For this review, take the finished solid that the model builds, in its own axes (mm). Face numbers are marked on the shaded views. A direction names the side the tool comes from. Round coordinates to 2 decimals unless told otherwise and drop trailing zeros. Order: outer loops, then holes, each group sorted by start corner. A loop starts at its lowest first (then second) coordinate and runs counter-clockwise, first axis right, second up. Notation, with made-up numbers: (21, -7) -> (36, -7) arc R15 ccw to (36, 16) -> close; hole circle Ø5 at (35, 68.5). An arc over 180 degrees is marked (long way). Answer in a Markdown table with one row per item.
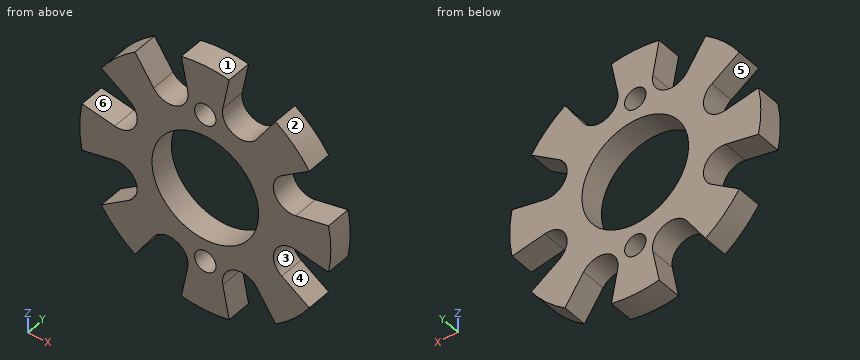
```python
from build123d import *

# Parameters (mm, degrees)
SKETCH1_R           = 20
BOSS_EXTRUDE1_DEPTH = 4
CUT_EXTRUDE1_REACH  = 6
SKETCH2_R           = 4
SKETCH2_R_2         = 1.7
CUT_EXTRUDE3_DEPTH  = 4
CIRPATTERN1_COUNT   = 8
SKETCH4_R           = 8.5
CUT_EXTRUDE4_DEPTH  = 5


with BuildPart() as part:
    # Sketch1 → Boss-Extrude1 (new body)
    with BuildSketch(Plane(origin=(0, 0, 0), x_dir=(1, 0, 0), z_dir=(0, 1, 0))):
        Circle(SKETCH1_R)
    extrude(amount=BOSS_EXTRUDE1_DEPTH)

    # Sketch2 → Cut-Extrude1 (cut, up to next)
    with BuildSketch(Plane(origin=(0, 0, 0), x_dir=(1, 0, 0), z_dir=(0, 1, 0)), mode=Mode.PRIVATE) as cut_extrude1_sk1:
        Circle(SKETCH2_R)
    cut_extrude1_tool1 = extrude(cut_extrude1_sk1.sketch, amount=CUT_EXTRUDE1_REACH, mode=Mode.PRIVATE) & part.part
    add(cut_extrude1_tool1.solids().sort_by_distance((0, 0, 0))[0], mode=Mode.SUBTRACT)
    # Sketch2 → Cut-Extrude1 (cut, up to next)
    with BuildSketch(Plane(origin=(0, 0, 0), x_dir=(1, 0, 0), z_dir=(0, 1, 0)), mode=Mode.PRIVATE) as cut_extrude1_sk2:
        with Locations((0, 12)):
            Circle(SKETCH2_R_2)
    cut_extrude1_tool2 = extrude(cut_extrude1_sk2.sketch, amount=CUT_EXTRUDE1_REACH, mode=Mode.PRIVATE) & part.part
    add(cut_extrude1_tool2.solids().sort_by_distance((0, 0, -12))[0], mode=Mode.SUBTRACT)
    # Sketch2 → Cut-Extrude1 (cut, up to next)
    with BuildSketch(Plane(origin=(0, 0, 0), x_dir=(1, 0, 0), z_dir=(0, 1, 0)), mode=Mode.PRIVATE) as cut_extrude1_sk3:
        with Locations((0, -12)):
            Circle(SKETCH2_R_2)
    cut_extrude1_tool3 = extrude(cut_extrude1_sk3.sketch, amount=CUT_EXTRUDE1_REACH, mode=Mode.PRIVATE) & part.part
    add(cut_extrude1_tool3.solids().sort_by_distance((0, 0, 12))[0], mode=Mode.SUBTRACT)

    # Sketch3 → Cut-Extrude3 (cut)
    with BuildSketch(Plane(origin=(0, 0, 0), x_dir=(1, 0, 0), z_dir=(0, 1, 0))):
        with BuildLine():
            ThreePointArc((3.803515008, 19.635001237), (7.653668647, 18.47759065), (11.194551269, 16.573533778))
            Line((11.194551269, 16.573533778), (8.226281552, 12.179010297))
            ThreePointArc((8.226281552, 12.179010297), (4.592201188, 11.08655439), (2.7950013, 14.428720239))
            Line((2.7950013, 14.428720239), (3.803515008, 19.635001237))
        make_face()
    cut_extrude3 = extrude(amount=CUT_EXTRUDE3_DEPTH, mode=Mode.SUBTRACT)

    # CirPattern1: Cut-Extrude3 ×8 about axis
    cirpattern1_axis = Axis((0, 0, 0), (0, 1, 0))
    for i in range(1, CIRPATTERN1_COUNT):
        add(cut_extrude3.rotate(cirpattern1_axis, i * 360 / CIRPATTERN1_COUNT), mode=Mode.SUBTRACT)

    # Sketch4 → Cut-Extrude4 (cut, through all)
    with BuildSketch(Plane(origin=(0, 4, 0), x_dir=(1, 0, 0), z_dir=(0, 1, 0))):
        Circle(SKETCH4_R)
    extrude(amount=-CUT_EXTRUDE4_DEPTH, mode=Mode.SUBTRACT)


solid = part.part
```
Q1. Take a section at C-C, the plane z = -15.5. Write out the cut boundary in (x, y).
Answer key:
| item | result |
|---|---|
| outline | (-12.64, 0) -> (-10.47, 0) -> (-10.47, 4) -> (-12.64, 4) -> close; (-3, 0) -> (3, 0) -> (3, 4) -> (-3, 4) -> close; (10.47, 0) -> (12.64, 0) -> (12.64, 4) -> (10.47, 4) -> close |
Q2. To check wall thickness, follow probe 1 along Z at (x, y) = (0, 2.8); probe 2 along X at (y, z) = (1.1, 0); probe 3 along X at (y, z) = (0.5, 11.5). State the ranges of each line that lie inside material, in increasing order.
Answer key:
| item | result |
|---|---|
| probe 1 | z = -20 to -13.7, -10.3 to -8.5, 8.5 to 10.3, 13.7 to 20 |
| probe 2 | x = -20 to -8.5, 8.5 to 20 |
| probe 3 | x = -16.36 to -7.59, -3.89 to -1.62, 1.62 to 3.89, 7.59 to 16.36 |
Q3. The part is to be moulded in two halves that separate along X. For the marked faces 1, 2 and 3, say which applies: +X half, -X half, draft (parallel to the pull), parting line (faces both ways), or undercut.
Answer key:
| item | result |
|---|---|
| face 1 | parting line |
| face 2 | +X half |
| face 3 | undercut |
Q4. Take a section at A-A, the plane x = 0. Write out the cut boundary in (y, z).
Answer key:
| item | result |
|---|---|
| outline | (0, -20) -> (4, -20) -> (4, -13.7) -> (0, -13.7) -> close; (0, -10.3) -> (4, -10.3) -> (4, -8.5) -> (0, -8.5) -> close; (0, 8.5) -> (4, 8.5) -> (4, 10.3) -> (0, 10.3) -> close; (0, 13.7) -> (4, 13.7) -> (4, 20) -> (0, 20) -> close |
Q5. Tool access review of the marked faces 4, 5 and 6: name each direction out of +Z, -Z, +X, -X, +Y, -Y from which nothing blocks a thin tool from reaching the whole face with its end or side.
Answer key:
| item | result |
|---|---|
| face 4 | +X, +Y, -Y |
| face 5 | -X, +Y, -Y |
| face 6 | +Y, -Y |
Q6. Take a section at B-B, the plane z = 0. Write out the cut boundary in (x, y).
Answer key:
| item | result |
|---|---|
| outline | (-20, 0) -> (-8.5, 0) -> (-8.5, 4) -> (-20, 4) -> close; (8.5, 0) -> (20, 0) -> (20, 4) -> (8.5, 4) -> close |
Q7. Clearance check with flat-ended pins moving along their axes: pin 1 Ø19.5 at (x, z) = (0, 0) entering from +Y; pin 2 Ø1.5 at (x, y) = (15.5, 1) entering from -Z. State where each tip first meets the part, or that it passes through.
Answer key:
| item | result |
|---|---|
| pin 1 | stops at y = 4 |
| pin 2 | stops at z = -13.51 |
Q8. Take a section at D-D, the plane x = 7.5. Write out the cut boundary in (y, z), then the cut area to 3 significant figures.
Answer key:
| item | result |
|---|---|
| outline | (0, -11.43) -> (4, -11.43) -> (4, -4) -> (0, -4) -> close; (0, 4) -> (4, 4) -> (4, 11.43) -> (0, 11.43) -> close |
| area | 59.4 mm^2 |
